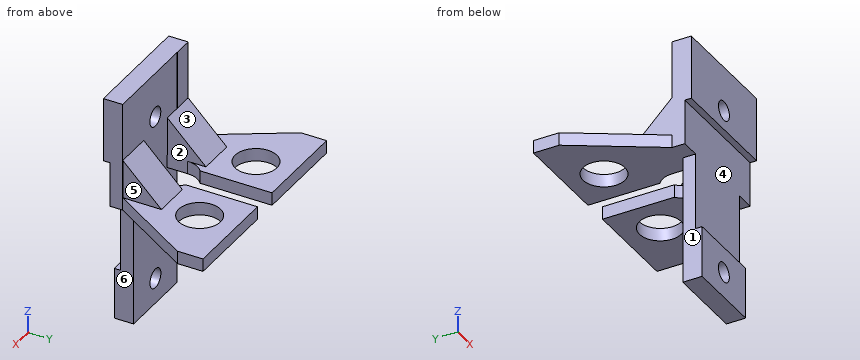
```python
from build123d import *

# Parameters (mm, degrees)
BOX_W           = 34
BOX_H           = 17
BOX_DEPTH       = 2
SKETCH_R        = 3.25
POCKET_DEPTH    = 2
SKETCH001_W     = 6.4987877113
SKETCH001_H     = 3.187234
POCKET001_DEPTH = 2
POCKET002_DEPTH = 2
SKETCH003_W     = 12
SKETCH003_H     = 2
PAD_DEPTH       = 2
SKETCH004_W     = 12
SKETCH004_H     = 2
PAD001_DEPTH    = 15
SKETCH005_W     = 12
SKETCH005_H     = 2
PAD002_DEPTH    = 20
SKETCH006_W     = 2.977736
SKETCH006_H     = 2.018581
SKETCH006_W_2   = 3
SKETCH006_H_2   = 2
PAD003_DEPTH    = 17
SKETCH007_W     = 17.977736
SKETCH007_H     = 10
SKETCH007_W_2   = 12
SKETCH007_H_2   = 8
PAD004_DEPTH    = 1
SKETCH008_R     = 1.5
POCKET003_DEPTH = 3
SKETCH009_W     = 4
SKETCH009_H     = 13.706681
POCKET004_DEPTH = 2
PAD005_DEPTH    = 5.7283421443
PAD006_DEPTH    = 5.7506061443


with BuildPart() as part:
    # Box → Box (new body)
    with BuildSketch(Plane.XY):
        with Locations((17, 8.5)):
            Rectangle(BOX_W, BOX_H)
    extrude(amount=BOX_DEPTH)

    # Sketch → Pocket (cut)
    with BuildSketch(Plane.XY.offset(2)):
        with Locations((9.25, 11.25)):
            Circle(SKETCH_R)
        with Locations((24.75, 11.25)):
            Circle(SKETCH_R)
        with Locations((17, 3.25)):
            Circle(SKETCH_R)
    extrude(amount=-POCKET_DEPTH, mode=Mode.SUBTRACT)

    # Sketch001 → Pocket001 (cut)
    with BuildSketch(Plane.XY.offset(2)):
        with Locations((17, 1.593617)):
            Rectangle(SKETCH001_W, SKETCH001_H)
    extrude(amount=-POCKET001_DEPTH, mode=Mode.SUBTRACT)

    # Sketch002 → Pocket002 (cut)
    with BuildSketch(Plane.XY.offset(2)):
        Polygon((0, 0), (8, 0), (0, 13), align=None)
        Polygon((34, 0), (26, 0), (34, 13), align=None)
    extrude(amount=-POCKET002_DEPTH, mode=Mode.SUBTRACT)

    # Sketch003 → Pad (new body)
    with BuildSketch(Plane.XZ):
        with Locations((17, 1)):
            Rectangle(SKETCH003_W, SKETCH003_H)
    extrude(amount=PAD_DEPTH)

    # Sketch004 → Pad001 (new body)
    with BuildSketch(Plane.XY.offset(2)):
        with Locations((17, -1)):
            Rectangle(SKETCH004_W, SKETCH004_H)
    extrude(amount=PAD001_DEPTH)

    # Sketch005 → Pad002 (new body)
    with BuildSketch(Plane(origin=(0, 0, 0), x_dir=(1, 0, 0), z_dir=(0, 0, -1))):
        with Locations((17, 1)):
            Rectangle(SKETCH005_W, SKETCH005_H)
    extrude(amount=PAD002_DEPTH)

    # Sketch006 → Pad003 (new body)
    with BuildSketch(Plane(origin=(0, 0, 0), x_dir=(1, 0, 0), z_dir=(0, 0, -1))):
        with Locations((9.511132, 0.9907095)):
            Rectangle(SKETCH006_W, SKETCH006_H)
        with Locations((24.5, 1)):
            Rectangle(SKETCH006_W_2, SKETCH006_H_2)
    extrude(amount=-PAD003_DEPTH)

    # Sketch007 → Pad004 (new body)
    with BuildSketch(Plane.XZ.offset(2)):
        with Locations((17.011132, 12)):
            Rectangle(SKETCH007_W, SKETCH007_H)
        with Locations((17, -16)):
            Rectangle(SKETCH007_W_2, SKETCH007_H_2)
    extrude(amount=PAD004_DEPTH)

    # Sketch008 → Pocket003 (cut)
    with BuildSketch(Plane.XZ.offset(3)):
        with Locations((17.022264, 10)):
            Circle(SKETCH008_R)
        with Locations((17, -16)):
            Circle(SKETCH008_R)
    extrude(amount=-POCKET003_DEPTH, mode=Mode.SUBTRACT)

    # Sketch009 → Pocket004 (cut)
    with BuildSketch(Plane.XY.offset(2)):
        with Locations((17, 10.5939175)):
            Rectangle(SKETCH009_W, SKETCH009_H)
    extrude(amount=-POCKET004_DEPTH, mode=Mode.SUBTRACT)

    # Sketch010 → Pad005 (new body)
    with BuildSketch(Plane(origin=(8.022264, 0, 0), x_dir=(0, -1, 0), z_dir=(-1, 0, 0))):
        Polygon((-0.018581, 2), (-6.018581, 2), (-0.018581, 8), align=None)
    extrude(amount=-PAD005_DEPTH)

    # Sketch011 → Pad006 (new body)
    with BuildSketch(Plane.YZ.offset(26)):
        Polygon((0.018581, 8), (0.018581, 2), (6.018581, 2), align=None)
    extrude(amount=-PAD006_DEPTH)


solid = part.part
```
Could you check a few things on this model? Use its own coordinates, in mm. Face numbers are marked on the shaded views. A direction names the side the tool comes from. Round coordinates to 2 decimals unless told otherwise and drop trailing zeros. Loops run counter-clockwise (first coordinate to the right, second up) from the corner with the lowest first, then second, coordinate; pieces in that order, holes last. Notation, with made-up numbers: M 89.5,29.5 L 96.5,29.5 A18 cw 96.5,38.5 Z; hole C 71.25,14.25 d11. An arc over 180 degrees is marked long. Put each result on its own line as item: value.
Q1. Imagine slicing it at D-D (y = 11.25). Write out the boundary of the cut face in (x, z).
Check result:
outline: M 1.08,0 L 6,0 L 6,2 L 1.08,2 Z; M 12.5,0 L 15,0 L 15,2 L 12.5,2 Z; M 19,0 L 21.5,0 L 21.5,2 L 19,2 Z; M 28,0 L 32.92,0 L 32.92,2 L 28,2 Z
Q2. Imagine slicing it at A-A (y = 15.75). Write out the boundary of the cut face in (x, z).
Check result:
outline: M 0,0 L 15,0 L 15,2 L 0,2 Z; M 19,0 L 34,0 L 34,2 L 19,2 Z
Q3. For pin 1 (8 mm diameter, centred on y = 1, z = 8.5, fed in from -X); pin 2 (6 mm diameter, centred on x = 24.75, y = 11.25, fed in from -Z); pin 3 (2 mm diameter, centred on x = 12.5, z = 5.5, fed in from -Y); pin 4 (1.5 mm diameter, centred on x = 9, z = 11, fed in from +Y), each with a flat end and sliding along its axis, tell me the tip position at first contact or that it passes through.
Check result:
pin 1: x = 8.02
pin 2: through
pin 3: y = -2
pin 4: y = 0.02
Q4. On a 3-axis mill with a long thin cutter (end or side, diameter ignored), from which of +Z, -Z, +X, -X, +Y, -Y can I reach the whole of each face in a straight line? I mean the marked faces 4, 5 and 6. Say none if no direction works.
Check result:
face 4: +X, -X, -Y
face 5: +Z, +X, +Y, -Y
face 6: -Z, +X, +Y, -Y
Q5. I need wall thicknesses on probe 1 along Z at (x, y) = (17, -0.95); probe 2 along Y at (x, z) = (9.25, 1.4); probe 3 along Y at (x, z) = (21.5, -10.5). Which ranges of each line are inside material? Lowest first, please.
Check result:
probe 1: -20 to -17.5, -14.5 to 8.5, 11.5 to 17
probe 2: -2 to 8, 14.5 to 17
probe 3: -2 to 0
Q6. Thinking about a two-plate mould opening in X: for the marked faces 1, 2 and 3, which applies, released by +X, released by -X, zero draft, split by the parting line, or undercut?
Check result:
face 1: released by -X
face 2: undercut
face 3: zero draft
